Print and shaded views of the part. All mm, measured from the part's lowest x, y and z. A direction names the side the tool comes from. Round coordinates to 2 decimals unless told otherwise and drop trailing zeros. Order: outer loops, then holes, each group sorted by start corner. A loop starts at its lowest first (then second) coordinate and runs counter-clockwise, first axis right, second up. Notation, with made-up numbers: (-22, 27.25) - (25, 27.25) arc R17 ccw to (25, 59.25) - close; hole circle Ø3 at (-33, -6). An arc over 180 degrees is marked (long way). Write item = value, one per line.
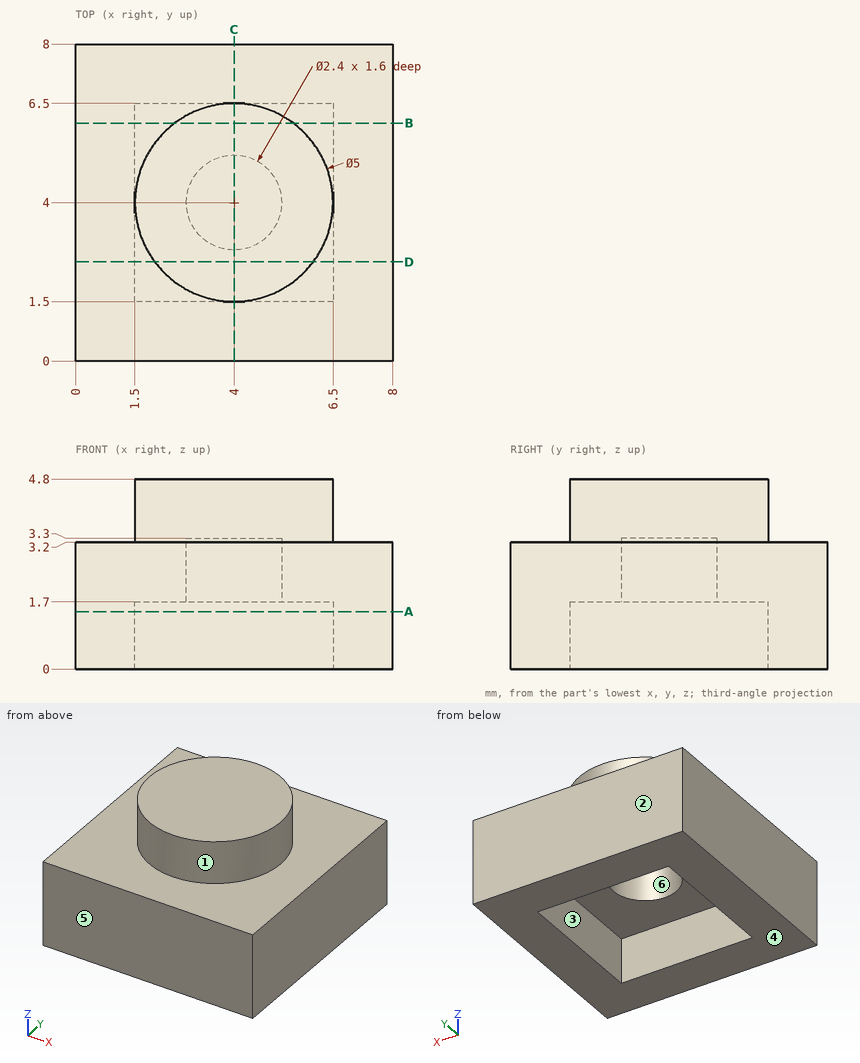
(1) Band-saw the part on B-B on y = 6. List the corners of the cut face in (x, z), plus the area to 3 significant figures.
Solved:
outline = (0, 0) - (1.5, 0) - (1.5, 1.7) - (6.5, 1.7) - (6.5, 0) - (8, 0) - (8, 3.2) - (5.5, 3.2) - (5.5, 4.8) - (2.5, 4.8) - (2.5, 3.2) - (0, 3.2) - close
area = 21.9 mm²
(2) Drop flat-ended pins along their axis: pin 1 (1.5 mm diameter, centred on y = 4, z = 3, fed in from -X); pin 2 (1.9 mm diameter, centred on x = 4, y = 4, fed in from -Z); pin 3 (2.5 mm diameter, centred on x = 4, y = 3.5, fed in from -Z). Give the stop position or say it passes through.
Solved:
pin_1 = 0
pin_2 = 3.3
pin_3 = 1.7
(3) Band-saw the part on A-A on z = 1.45. List the corners of the cut face in (x, y), plus the area to 3 significant figures.
Solved:
outline = (0, 0) - (8, 0) - (8, 8) - (0, 8) - close; hole (1.5, 1.5) - (6.5, 1.5) - (6.5, 6.5) - (1.5, 6.5) - close
area = 39.0 mm²
(4) Probe line 1 along X through (y, z) = (4.5, 1.3); line 2 along Y through (x, z) = (4, 2.8). List the from-to ranges inside material, lowest first.
Solved:
line_1 = 0 to 1.5, 6.5 to 8
line_2 = 0 to 2.8, 5.2 to 8
(5) Pull direction Y, two halves, no side cores. Call the marked faces 4, 5 and 6: released by +Y, released by -Y, zero draft, split by the parting line, or undercut.
Solved:
face_4 = zero draft
face_5 = released by -Y
face_6 = undercut
(6) Tool access for the marked faces 1, 2 and 3: list every direction of +Z, -Z, +X, -X, +Y, -Y with a clear straight run to the whole face (end or side of a thin tool).
Solved:
face_1 = +Z
face_2 = +Z, -Z, +X, -X, +Y
face_3 = -Z
(7) Band-saw the part on C-C on x = 4. List the corners of the cut face in (y, z).
Solved:
outline = (0, 0) - (1.5, 0) - (1.5, 1.7) - (2.8, 1.7) - (2.8, 3.3) - (5.2, 3.3) - (5.2, 1.7) - (6.5, 1.7) - (6.5, 0) - (8, 0) - (8, 3.2) - (6.5, 3.2) - (6.5, 4.8) - (1.5, 4.8) - (1.5, 3.2) - (0, 3.2) - close
(8) Band-saw the part on D-D on y = 2.5. List the corners of the cut face in (x, z), plus the area to 3 significant figures.
Solved:
outline = (0, 0) - (1.5, 0) - (1.5, 1.7) - (6.5, 1.7) - (6.5, 0) - (8, 0) - (8, 3.2) - (6, 3.2) - (6, 4.8) - (2, 4.8) - (2, 3.2) - (0, 3.2) - close
area = 23.5 mm²
